Part print with two shaded views. Sizes in mm from the minimum x, y, z corner. A direction names the side the tool comes from. Coordinates: 2 decimals unless noted, no trailing zeros. Order: outer loops, then holes, each group sorted by start corner. A loop starts at its lowest first (then second) coordinate and runs counter-clockwise, first axis right, second up.
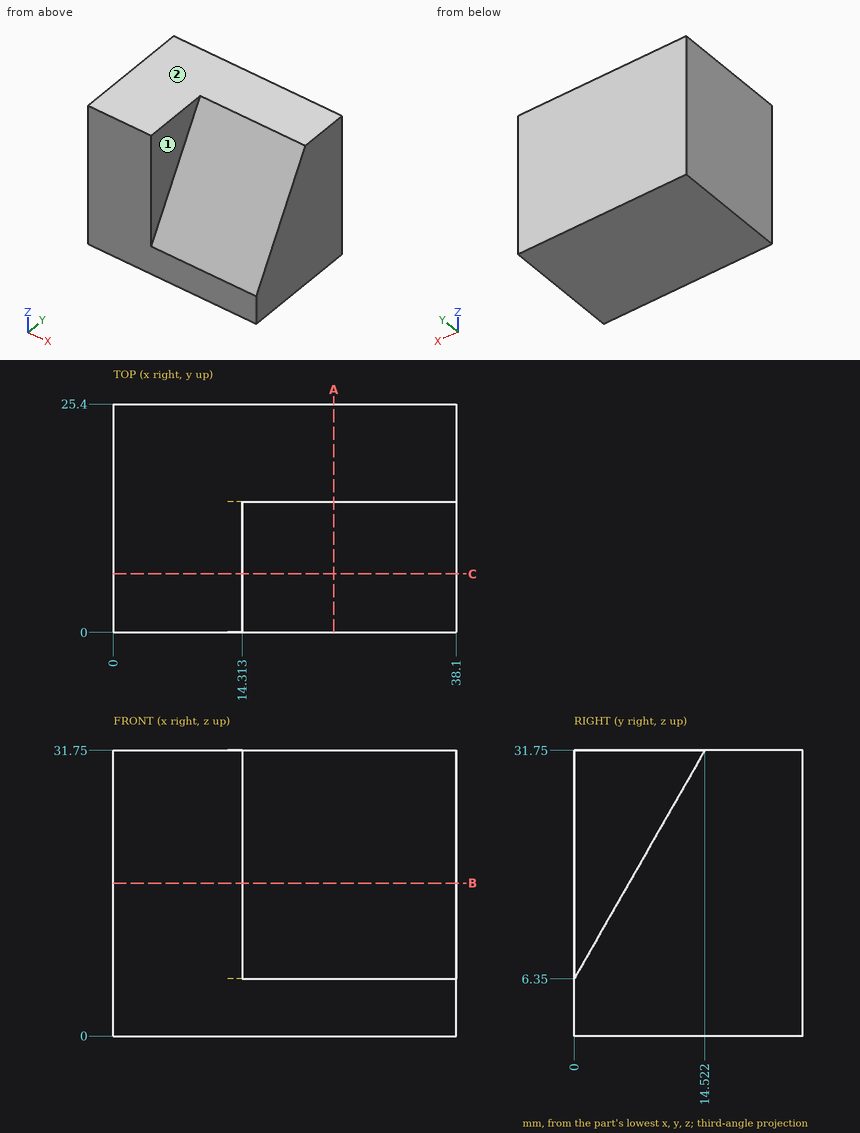
Q1. Which spindle directions (+Z, -Z, +X, -X, +Y, -Y) get a long thin tool onto all of the face, cutting with end or side? Do the marked faces 1 and 2. Say none if no direction does.
Results list:
face 1: +Z, +X, -Y
face 2: +Z, +X, -X, +Y, -Y
Q2. Wall check: line 1 along X through (y, z) = (4, 21); line 2 along Z through (x, y) = (31, 2.5) (1 decimal); line 3 along Y through (x, z) = (28, 8) (1 decimal). Give the ranges that are in metal, low to high.
Results list:
line 1: x = 0 to 14.31
line 2: z = 0 to 10.7
line 3: y = 0.9 to 25.4
Q3. Cut at A-A on x = 24.5. Write the cut outline in (y, z).
Results list:
outline: (0, 0) - (25.4, 0) - (25.4, 31.75) - (14.52, 31.75) - (0, 6.35) - close
Q4. Cut at C-C on y = 6.5. Write the cut outline in (x, z).
Results list:
outline: (0, 0) - (38.1, 0) - (38.1, 17.72) - (14.31, 17.72) - (14.31, 31.75) - (0, 31.75) - close
Q5. Cut at B-B on z = 17. Write the cut outline in (x, y), and give its area (3 significant figures).
Results list:
outline: (0, 0) - (14.31, 0) - (14.31, 6.09) - (38.1, 6.09) - (38.1, 25.4) - (0, 25.4) - close
area: 823 mm2
